```python
from build123d import *

# Parameters (mm, degrees)
SKETCH_1_W            = 16.5
SKETCH_1_H            = 10
SKETCH_1_W_2          = 1
SKETCH_1_H_2          = 92
CUT_EXTRUDE_START     = -10
SKETCH_2_W            = 1.7
SKETCH_2_H            = 2
CUT_EXTRUDE_1_DEPTH   = 10
EXTRUDE_START         = -250
SKETCH_3_R            = 50
SKETCH_3_R_2          = 32.5
EXTRUDE_1_DEPTH       = 250
EXTRUDE_7_DEPTH       = 250
EXTRUDE_8_DEPTH       = 50
EXTRUDE_8_DEPTH_BACK  = 50
CUT_EXTRUDE_2_DEPTH   = 9.525
SKETCH_7_W            = 44.95012806
SKETCH_7_H            = 44.95012806
CUT_EXTRUDE_3_DEPTH   = 33
SKETCH_12_W           = 100
SKETCH_12_H           = 500
EXTRUDE_10_DEPTH      = 239
EXTRUDE_12_DEPTH      = 73
EXTRUDE_12_DEPTH_BACK = 612
SKETCH_13_R           = 15


with BuildPart() as part:
    # Sketch 1 → Revolve 1 (revolve)
    with BuildSketch(Plane.XY, mode=Mode.PRIVATE) as revolve_1_sk:
        Polygon((-10, 0), (0, 0), (0, 10), (0, 102), (0, 250), (-10, 250), align=None)
        with Locations((8.25, 5)):
            Rectangle(SKETCH_1_W, SKETCH_1_H)
        with Locations((36.75, 5)):
            Rectangle(SKETCH_1_W, SKETCH_1_H)
        with Locations((44.5, 56)):
            Rectangle(SKETCH_1_W_2, SKETCH_1_H_2)
        Polygon((45, 10), (45, 0), (55, 0), (55, 250), (45, 250), (45, 102), align=None)
        with Locations((0.5, 56)):
            Rectangle(SKETCH_1_W_2, SKETCH_1_H_2)
    revolve(revolve_1_sk.sketch.rotate(Axis((22.5, 0, 0), (0, 1, 0)), 270), axis=Axis((22.5, 0, 0), (0, 1, 0)))

    # Sketch 2 → Cut-Extrude 1 (cut)
    with BuildSketch(Plane.XZ.offset(CUT_EXTRUDE_START)):
        with Locations((29.35, -1)):
            Rectangle(SKETCH_2_W, SKETCH_2_H)
        with BuildLine():
            Line((28.5, -2), (28.5, 0))
            ThreePointArc((28.5, 0), (28.413591358, -1.014611872), (28.156854249, -2))
            Line((28.156854249, -2), (28.5, -2))
        make_face()
        with BuildLine():
            ThreePointArc((28.156854249, 2), (28.413591358, 1.014611872), (28.5, 0))
            Line((28.5, 0), (28.5, 2))
            Line((28.5, 2), (28.156854249, 2))
        make_face()
        with Locations((29.35, 1)):
            Rectangle(SKETCH_2_W, SKETCH_2_H)
    extrude(amount=CUT_EXTRUDE_1_DEPTH, mode=Mode.SUBTRACT)

    # Sketch 3 → Extrude 1 (add)
    with BuildSketch(Plane(origin=(0, 250, 0), x_dir=(1, 0, 0), z_dir=(0, 1, 0)).offset(EXTRUDE_START)):
        with Locations(Location((22.5, 0, 0), (0, 0, 270))):
            Circle(SKETCH_3_R)
        with Locations((22.5, 0)):
            Circle(SKETCH_3_R_2, mode=Mode.SUBTRACT)
    extrude(amount=EXTRUDE_1_DEPTH)

    # Sketch 3_5 → Extrude 7 (add)
    with BuildSketch(Plane(origin=(0, 250, 0), x_dir=(1, 0, 0), z_dir=(0, 1, 0)).offset(EXTRUDE_START)):
        with BuildLine():
            ThreePointArc((72.5, 0), (57.855339059, -35.355339059), (22.5, -50))
            Line((22.5, -50), (72.5, -50))
            Line((72.5, -50), (72.5, 0))
        make_face()
        with BuildLine():
            ThreePointArc((22.5, -50), (-12.855339059, -35.355339059), (-27.5, 0))
            Line((-27.5, 0), (-27.5, -50))
            Line((-27.5, -50), (22.5, -50))
        make_face()
        with BuildLine():
            Line((72.5, 50), (22.5, 50))
            ThreePointArc((22.5, 50), (57.855339059, 35.355339059), (72.5, 0))
            Line((72.5, 0), (72.5, 50))
        make_face()
        with BuildLine():
            Line((-27.5, 50), (-27.5, 0))
            ThreePointArc((-27.5, 0), (-12.855339059, 35.355339059), (22.5, 50))
            Line((22.5, 50), (-27.5, 50))
        make_face()
    extrude(amount=EXTRUDE_7_DEPTH)

    # Sketch 1_21 → Extrude 8 (add, two sides: drawn at the far end of the back side and taken through both)
    with BuildSketch(Plane.XY.offset(-EXTRUDE_8_DEPTH_BACK)):
        Polygon((16.5, 0), (0, 0), (-10, 0), (-27.5, 0), (-27.5, -33), (72.5, -33), (72.5, 0), (55, 0), (45, 0), (28.5, 0), align=None)
    extrude(amount=EXTRUDE_8_DEPTH + EXTRUDE_8_DEPTH_BACK)

    # Sketch 5 → Cut-Extrude 2 (cut)
    with BuildSketch(Plane.XZ.offset(33)):
        with BuildLine():
            ThreePointArc((0.02493597, -27.24506403), (-0.33815866, -25.419664058), (-1.372164684, -23.872164684))
            Line((-1.372164684, -23.872164684), (-8.117963377, -30.617963377))
            ThreePointArc((-8.117963377, -30.617963377), (-2.919664058, -31.6519694), (0.02493597, -27.24506403))
        make_face()
        with BuildLine():
            Line((-8.117963377, -30.617963377), (-1.372164684, -23.872164684))
            ThreePointArc((-1.372164684, -23.872164684), (-8.117963377, -23.872164684), (-8.117963377, -30.617963377))
        make_face()
        with BuildLine():
            ThreePointArc((27.27, -38.530339059), (25.872899346, -35.157439713), (22.5, -33.760339059))
            Line((22.5, -33.760339059), (22.5, -43.300339059))
            ThreePointArc((22.5, -43.300339059), (25.872899346, -41.903238406), (27.27, -38.530339059))
        make_face()
        with BuildLine():
            Line((22.5, -43.300339059), (22.5, -33.760339059))
            ThreePointArc((22.5, -33.760339059), (17.73, -38.530339059), (22.5, -43.300339059))
        make_face()
        with BuildLine():
            ThreePointArc((54.51506403, -27.24506403), (51.570464003, -22.83815866), (46.372164684, -23.872164684))
            Line((46.372164684, -23.872164684), (53.117963377, -30.617963377))
            ThreePointArc((53.117963377, -30.617963377), (54.1519694, -29.070464003), (54.51506403, -27.24506403))
        make_face()
        with BuildLine():
            Line((53.117963377, -30.617963377), (46.372164684, -23.872164684))
            ThreePointArc((46.372164684, -23.872164684), (46.372164684, -30.617963377), (53.117963377, -30.617963377))
        make_face()
        with BuildLine():
            ThreePointArc((65.800339059, 0), (61.030339059, 4.77), (56.260339059, 0))
            Line((56.260339059, 0), (65.800339059, 0))
        make_face()
        with BuildLine():
            Line((65.800339059, 0), (56.260339059, 0))
            ThreePointArc((56.260339059, 0), (61.030339059, -4.77), (65.800339059, 0))
        make_face()
        with BuildLine():
            ThreePointArc((53.117963377, 30.617963377), (46.372164684, 30.617963377), (46.372164684, 23.872164684))
            Line((46.372164684, 23.872164684), (53.117963377, 30.617963377))
        make_face()
        with BuildLine():
            Line((53.117963377, 30.617963377), (46.372164684, 23.872164684))
            ThreePointArc((46.372164684, 23.872164684), (51.570464003, 22.83815866), (54.51506403, 27.24506403))
            ThreePointArc((54.51506403, 27.24506403), (54.1519694, 29.070464003), (53.117963377, 30.617963377))
        make_face()
        with BuildLine():
            ThreePointArc((22.5, 43.300339059), (17.73, 38.530339059), (22.5, 33.760339059))
            Line((22.5, 33.760339059), (22.5, 43.300339059))
        make_face()
        with BuildLine():
            Line((22.5, 43.300339059), (22.5, 33.760339059))
            ThreePointArc((22.5, 33.760339059), (25.872899346, 35.157439713), (27.27, 38.530339059))
            ThreePointArc((27.27, 38.530339059), (25.872899346, 41.903238406), (22.5, 43.300339059))
        make_face()
        with BuildLine():
            ThreePointArc((-8.117963377, 30.617963377), (-8.117963377, 23.872164684), (-1.372164684, 23.872164684))
            Line((-1.372164684, 23.872164684), (-2.5, 25))
            Line((-2.5, 25), (-6.990128061, 29.490128061))
            Line((-6.990128061, 29.490128061), (-8.117963377, 30.617963377))
        make_face()
        with BuildLine():
            Line((-2.5, 25), (-1.372164684, 23.872164684))
            ThreePointArc((-1.372164684, 23.872164684), (-0.33815866, 25.419664058), (0.02493597, 27.24506403))
            ThreePointArc((0.02493597, 27.24506403), (-2.919664058, 31.6519694), (-8.117963377, 30.617963377))
            Line((-8.117963377, 30.617963377), (-6.990128061, 29.490128061))
            Line((-6.990128061, 29.490128061), (-2.5, 25))
        make_face()
        with BuildLine():
            ThreePointArc((-11.260339059, 0), (-16.030339059, 4.77), (-20.800339059, 0))
            Line((-20.800339059, 0), (-11.260339059, 0))
        make_face()
        with BuildLine():
            Line((-11.260339059, 0), (-20.800339059, 0))
            ThreePointArc((-20.800339059, 0), (-16.030339059, -4.77), (-11.260339059, 0))
        make_face()
    extrude(amount=-CUT_EXTRUDE_2_DEPTH, mode=Mode.SUBTRACT)

    # Sketch 7 → Cut-Extrude 3 (cut)
    with BuildSketch(Plane.XZ.offset(33)):
        with Locations((22.5, 0)):
            Rectangle(SKETCH_7_W, SKETCH_7_H)
    extrude(amount=-CUT_EXTRUDE_3_DEPTH, mode=Mode.SUBTRACT)

    # Sketch 12 → Extrude 10 (add)
    with BuildSketch(Plane(origin=(0, 0, -50), x_dir=(-1, 0, 0), z_dir=(0, 0, -1))):
        with Locations((-22.5, 217)):
            Rectangle(SKETCH_12_W, SKETCH_12_H)
    extrude(amount=EXTRUDE_10_DEPTH)

    # Sketch 13 → Extrude 12 (add, two sides: drawn at the far end of the back side and taken through both)
    with BuildSketch(Plane(origin=(0, 467, 0), x_dir=(1, 0, 0), z_dir=(0, 1, 0)).offset(-EXTRUDE_12_DEPTH_BACK)):
        with Locations(Location((22.5, 150, 0), (0, 0, 90))):
            Circle(SKETCH_13_R)
    extrude(amount=EXTRUDE_12_DEPTH + EXTRUDE_12_DEPTH_BACK)


solid = part.part
```
The model under review builds one solid part; all positions refer to its coordinate system, in mm. A direction names the side the tool comes from. Coordinates: 2 decimals unless noted, no trailing zeros. Write each loop counter-clockwise with the first axis right and the second up, starting at its lowest first coordinate (ties: lowest second). Pieces come first, ordered by that corner, then holes. Notation, with made-up numbers: (63.25, 69) - (103.25, 69) arc R18 cw to (103.25, 96) - close; hole circle Ø4 at (68, -14.5). An arc over 180 degrees is marked (long way). Answer in a Markdown table with one row per item. Add a question column.
Q1. Clearance check with flat-ended pins moving along their axes: pin 1 (5 mm diameter, centred on x = 0.5, y = 302.5, fed in from +Z); pin 2 (5 mm diameter, centred on x = -16.5, z = 2, fed in from -Y) (3 decimals); pin 3 (5 mm diameter, centred on x = 18.5, z = -192, fed in from +Y); pin 4 (10 mm diameter, centred on x = 27, z = -165, fed in from -Y). State where each tip first meets the part, or that it passes through.
Q2. For faces 4 (the face through (18, 10, -4.5)), 5 (the face through (44.975, -17, 0)), 6 (the face through (22, 110, 50)), list the 3-axis set-ups (+Z, -Z, +X, -X, +Y, -Y) from which the entire face can be reached by the end or side of a thin tool; tool diameter is ignored.
Q3. Consider section C-C on y = -83.5. Give the boundary of the cut face in (x, z).
Q4. Consider section D-D on z = -195. Give the boundary of the cut face in (x, y).
Q5. Draft analysis for pull direction Z (two halves, no side actions). For faces 1 (the face through (23, 360, -50)), 2 (the face through (22, 250, -23)), 3 (the face through (22, -17, 22.475)), state which applies: +Z half, -Z half, draft (parallel to the pull), parting line (faces both ways), or undercut.
Q6. To check wall thickness, follow line 1 along X through (y, z) = (-28.5, 0); line 2 along Z through (x, y) = (22.5, 5); line 3 along Z through (x, y) = (22, 131). State the ranges of each line that lie inside material, in increasing order. Write a range as from..to.
Q7. Consider section B-B on y = 142. Give the boundary of the cut face in (x, z), then the cut area to 3 significant figures.
Q8. Consider section A-A on z = -150. Give the boundary of the cut face in (x, y), then the cut area to 4 significant figures.
Answers below:
| question | item | result |
|---|---|---|
| 1 | pin 1 | z = -50 |
| 1 | pin 2 | y = -23.475 |
| 1 | pin 3 | y = 467 |
| 1 | pin 4 | y = -145 |
| 2 | face 4 | +Y |
| 2 | face 5 | -Y |
| 2 | face 6 | +Z, +X, -X, +Y, -Y |
| 3 | outline | circle Ø30 at (22.5, -150) |
| 4 | outline | (-27.5, -33) - (72.5, -33) - (72.5, 467) - (-27.5, 467) - close |
| 5 | face 1 | +Z half |
| 5 | face 2 | draft |
| 5 | face 3 | undercut |
| 6 | line 1 | -27.5..-20.8, -11.26..0.02, 44.98..56.26, 65.8..72.5 |
| 6 | line 2 | -289..-6, 6..50 |
| 6 | line 3 | -289..-22.49, 22.49..50 |
| 7 | outline | (-27.5, -289) - (72.5, -289) - (72.5, 50) - (-27.5, 50) - close; hole circle Ø45 at (22.5, 0) |
| 7 | area | 32,300 mm² |
| 8 | outline | (-27.5, -33) - (7.5, -33) - (7.5, -145) - (37.5, -145) - (37.5, -33) - (72.5, -33) - (72.5, 467) - (37.5, 467) - (37.5, 540) - (7.5, 540) - (7.5, 467) - (-27.5, 467) - close |
| 8 | area | 55,550 mm² |
